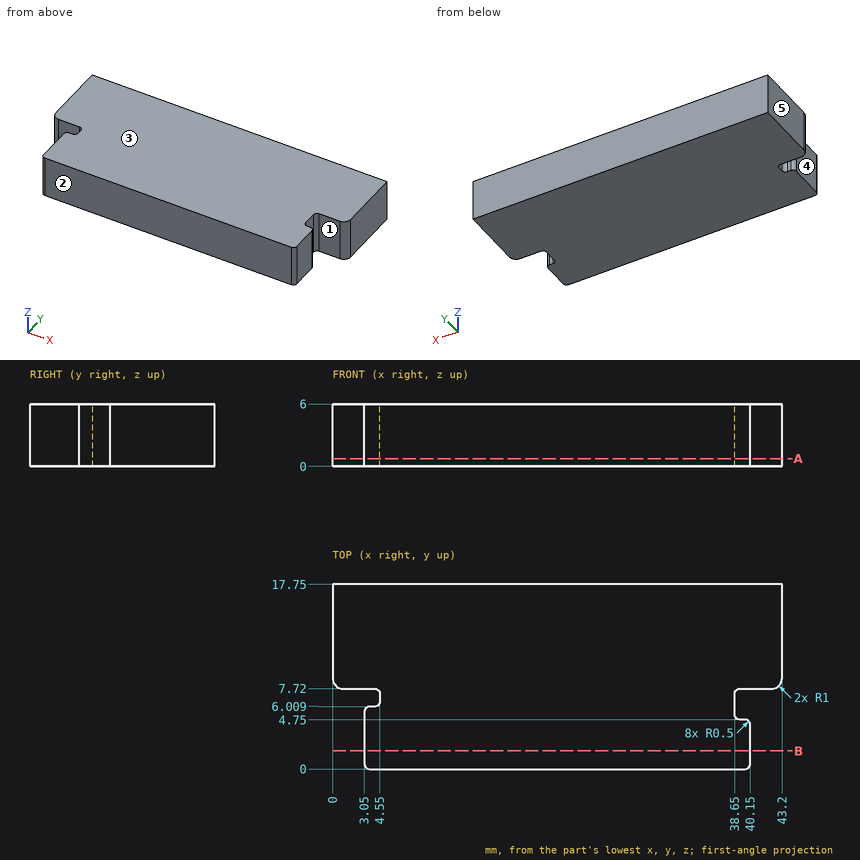
Geometry: see drawing. Coordinates: mm, zero at the bounding-box minimum. A direction names the side the tool comes from. Round coordinates to 2 decimals unless told otherwise and drop trailing zeros. Loops run counter-clockwise (first coordinate to the right, second up) from the corner with the lowest first, then second, coordinate; pieces in that order, holes last. Notation, with made-up numbers: (15, 34.25) -> (26, 34.25) arc R9 cw to (26, 48.25) -> close; hole circle Ø9 at (53, 84.25). An arc over 180 degrees is marked (long way). Write each question's results on one line, items separated by ' | '.
1. Section A-A (z = 0.75). Return loops of the section in (x, y), and give its area (3 significant figures).
Geometry results:
outline: (0, 8.72) arc R1 ccw to (1, 7.72) -> (4.05, 7.72) arc R0.5 cw to (4.55, 7.22) -> (4.55, 6.51) arc R0.5 cw to (4.05, 6.01) -> (3.55, 6.01) arc R0.5 ccw to (3.05, 5.51) -> (3.05, 0.5) arc R0.5 ccw to (3.55, 0) -> (39.65, 0) arc R0.5 ccw to (40.15, 0.5) -> (40.15, 4.25) arc R0.5 ccw to (39.65, 4.75) -> (39.15, 4.75) arc R0.5 cw to (38.65, 5.25) -> (38.65, 7.22) arc R0.5 cw to (39.15, 7.72) -> (42.2, 7.72) arc R1 ccw to (43.2, 8.72) -> (43.2, 17.75) -> (0, 17.75) -> close | area: 712 mm2
2. Mould query, pull axis Y, two halves, no side actions, for the marked faces 1, 2 and 3. Classes: +Y half, -Y half, draft (parallel to the pull), parting line (faces both ways), or undercut.
Geometry results:
face 1: undercut | face 2: -Y half | face 3: draft
3. Section B-B (y = 1.75). Return loops of the section in (x, z).
Geometry results:
outline: (3.05, 0) -> (40.15, 0) -> (40.15, 6) -> (3.05, 6) -> close
4. Set-up query: the marked faces 4 and 5. Return all of +Z, -Z, +X, -X, +Y, -Y with unobstructed straight access to the full face (end or side cutting, diameter ignored); none if empty.
Geometry results:
face 4: +Z, -Z, -X, -Y | face 5: +Z, -Z, -X, +Y, -Y
5. First-contact query: P1, Ø1.9, axis at y = 2, z = 2.5, coming from the +X side; P2, Ø1.5, axis at y = 5.5, z = 1.5, coming from the -X side; P3, Ø0.6, axis at y = 6.5, z = 4.5, coming from the +X side. Flat tips, straight axial feed; report the tip coordinate or a pass-through.
Geometry results:
P1: x = 40.15 | P2: x = 3.05 | P3: x = 38.65
6. Ray query, line 1 (X direction, y = 7, z = 2.7); line 2 (X direction, y = 1.5, z = 4.6). Return the intervals inside material, ascending. Write a range as from..to.
Geometry results:
line 1: 4.55..38.65 | line 2: 3.05..40.15
